Design review of the part built by this model. Coordinates are the model's own, in mm. Round coordinates to 2 decimals unless told otherwise and drop trailing zeros. One line per item, written item: value. Start each with the question number.
Item 1: For line 1 along Y through (x, z) = (-16.75, 168.5); line 2 along Y through (x, z) = (-12.7, 100.5); line 3 along X through (y, z) = (11, 50), list the stretches that pass through material, from the lowest coordinate up.
Item 2: Clearance check with flat-ended pins moving along their axes: pin 1 (3 mm diameter, centred on x = -12.5, z = 71, fed in from -Y); pin 2 (1.5 mm diameter, centred on y = 12, z = 160, fed in from +X); pin 3 (1.5 mm diameter, centred on y = 12.5, z = 79, fed in from -X). State where each tip first meets the part, or that it passes through.
Item 3: Mouldability with a two-part tool opening along X and no side actions: class faces 1 (the cylindrical face through (-1.086, 24.254, 106.439)), 2 (the cylindrical face through (-15.18, 14.97, 106.44)), 3 (the flat face through (-16, 16, 215.9)), 4 (the flat face through (-25.4, 19, 106)) as released by +X, released by -X, zero draft, split by the parting line, or undercut.
from build123d import *

# Parameters (mm, degrees)
F0_R     = 3.362501
F1_DEPTH = 215.9


with BuildPart() as f1:
    # F0 (on Top) → F1 (new body)
    with BuildSketch(Plane.XY):
        with BuildLine():
            ThreePointArc((-8.548576, 18.755238), (-9.784629, 17.929334), (-11.242653, 17.639315))
            Line((-11.242653, 17.639315), (-14.157347, 17.639315))
            ThreePointArc((-14.157347, 17.639315), (-15.615371, 17.929334), (-16.851424, 18.755238))
            Line((-16.851424, 18.755238), (-18.696905, 20.600719))
            ThreePointArc((-18.696905, 20.600719), (-19.109857, 22.67677), (-17.349867, 23.852758))
            Line((-17.349867, 23.852758), (-15.615371, 23.852758))
            Line((-15.615371, 23.852758), (-15.58302, 23.852758))
            ThreePointArc((-15.58302, 23.852758), (-14.825405, 24.626379), (-15.58302, 25.4))
            Line((-15.58302, 25.4), (-15.615371, 25.4))
            Line((-15.615371, 25.4), (-16.253341, 25.4))
            ThreePointArc((-16.253341, 25.4), (-16.801604, 24.858772), (-17.349867, 25.4))
            Line((-17.349867, 25.4), (-20.487482, 25.4))
            ThreePointArc((-20.487482, 25.4), (-21.038741, 24.848741), (-21.59, 25.4))
            ThreePointArc((-21.59, 25.4), (-24.284077, 24.284077), (-25.4, 21.59))
            Line((-25.4, 21.59), (-25.4, 20.504724))
            Line((-25.4, 20.504724), (-25.4, 17.349867))
            ThreePointArc((-25.4, 17.349867), (-24.844161, 16.802675), (-25.4, 16.255483))
            Line((-25.4, 16.255483), (-25.4, 15.615371))
            ThreePointArc((-25.4, 15.615371), (-24.626379, 14.859554), (-23.852758, 15.615371))
            Line((-23.852758, 15.615371), (-23.852758, 17.349867))
            ThreePointArc((-23.852758, 17.349867), (-22.67677, 19.109857), (-20.600719, 18.696905))
            Line((-20.600719, 18.696905), (-18.755238, 16.851424))
            ThreePointArc((-18.755238, 16.851424), (-17.929334, 15.615371), (-17.639315, 14.157347))
            Line((-17.639315, 14.157347), (-17.639315, 11.242653))
            ThreePointArc((-17.639315, 11.242653), (-17.929334, 9.784629), (-18.755238, 8.548576))
            Line((-18.755238, 8.548576), (-20.600719, 6.703095))
            ThreePointArc((-20.600719, 6.703095), (-22.67677, 6.290143), (-23.852758, 8.050133))
            Line((-23.852758, 8.050133), (-23.852758, 9.784629))
            ThreePointArc((-23.852758, 9.784629), (-24.626379, 10.55825), (-25.4, 9.784629))
            Line((-25.4, 9.784629), (-25.4, 9.149239))
            ThreePointArc((-25.4, 9.149239), (-24.899374, 8.599686), (-25.4, 8.050133))
            Line((-25.4, 8.050133), (-25.4, 4.904538))
            ThreePointArc((-25.4, 4.904538), (-24.846216, 4.357269), (-25.4, 3.81))
            ThreePointArc((-25.4, 3.81), (-24.284077, 1.115923), (-21.59, 0))
            ThreePointArc((-21.59, 0), (-21.040817, 0.554885), (-20.491634, 0))
            Line((-20.491634, 0), (-16.708169, 0))
            ThreePointArc((-16.708169, 0), (-16.16177, 0.540135), (-15.615371, 0))
            ThreePointArc((-15.615371, 0), (-14.854184, 0.7747), (-15.615371, 1.5494))
            Line((-15.615371, 1.5494), (-17.347709, 1.5494))
            ThreePointArc((-17.347709, 1.5494), (-19.107699, 2.725388), (-18.694747, 4.801438))
            Line((-18.694747, 4.801438), (-16.851424, 6.644762))
            ThreePointArc((-16.851424, 6.644762), (-15.615371, 7.470666), (-14.157347, 7.760685))
            Line((-14.157347, 7.760685), (-11.242653, 7.760685))
            ThreePointArc((-11.242653, 7.760685), (-9.784629, 7.470666), (-8.548576, 6.644762))
            Line((-8.548576, 6.644762), (-6.705253, 4.801438))
            ThreePointArc((-6.705253, 4.801438), (-6.292301, 2.725388), (-8.052291, 1.5494))
            Line((-8.052291, 1.5494), (-9.784629, 1.5494))
            ThreePointArc((-9.784629, 1.5494), (-10.401836, 0.7747), (-9.784629, 0))
            Line((-9.784629, 0), (-9.152868, 0))
            ThreePointArc((-9.152868, 0), (-8.602579, 0.545262), (-8.052291, 0))
            Line((-8.052291, 0), (-4.898866, 0))
            ThreePointArc((-4.898866, 0), (-4.354433, 0.544433), (-3.81, 0))
            ThreePointArc((-3.81, 0), (-1.115923, 1.115923), (0, 3.81))
            ThreePointArc((0, 3.81), (-0.53938, 4.3561), (0, 4.9022))
            Line((0, 4.9022), (0, 8.052291))
            ThreePointArc((0, 8.052291), (-0.543517, 8.60166), (0, 9.151029))
            Line((0, 9.151029), (0, 9.784629))
            ThreePointArc((0, 9.784629), (-0.7747, 10.504691), (-1.5494, 9.784629))
            Line((-1.5494, 9.784629), (-1.5494, 8.052291))
            ThreePointArc((-1.5494, 8.052291), (-2.725388, 6.292301), (-4.801438, 6.705253))
            Line((-4.801438, 6.705253), (-6.644762, 8.548576))
            ThreePointArc((-6.644762, 8.548576), (-7.470666, 9.784629), (-7.760685, 11.242653))
            Line((-7.760685, 11.242653), (-7.760685, 14.157347))
            ThreePointArc((-7.760685, 14.157347), (-7.470666, 15.615371), (-6.644762, 16.851424))
            Line((-6.644762, 16.851424), (-4.801438, 18.694747))
            ThreePointArc((-4.801438, 18.694747), (-2.725388, 19.107699), (-1.5494, 17.347709))
            Line((-1.5494, 17.347709), (-1.5494, 15.615371))
            ThreePointArc((-1.5494, 15.615371), (-0.7747, 14.879405), (0, 15.615371))
            Line((0, 15.615371), (0, 16.255509))
            ThreePointArc((0, 16.255509), (-0.5461, 16.801609), (0, 17.347709))
            Line((0, 17.347709), (0, 20.495165))
            ThreePointArc((0, 20.495165), (-0.551056, 21.042583), (0, 21.59))
            ThreePointArc((0, 21.59), (-1.115923, 24.284077), (-3.81, 25.4))
            ThreePointArc((-3.81, 25.4), (-4.365303, 24.903619), (-4.920606, 25.4))
            Line((-4.920606, 25.4), (-8.050133, 25.4))
            ThreePointArc((-8.050133, 25.4), (-8.596365, 24.859433), (-9.142596, 25.4))
            Line((-9.142596, 25.4), (-9.784629, 25.4))
            Line((-9.784629, 25.4), (-9.856203, 25.4))
            ThreePointArc((-9.856203, 25.4), (-10.594864, 24.626379), (-9.856203, 23.852758))
            Line((-9.856203, 23.852758), (-9.784629, 23.852758))
            Line((-9.784629, 23.852758), (-8.050133, 23.852758))
            ThreePointArc((-8.050133, 23.852758), (-6.290143, 22.67677), (-6.703095, 20.600719))
            Line((-6.703095, 20.600719), (-8.548576, 18.755238))
        make_face()
        with Locations((-12.7, 12.7)):
            Circle(F0_R, mode=Mode.SUBTRACT)
        with BuildLine():
            ThreePointArc((-9.856203, 23.852758), (-9.820416, 23.851931), (-9.784629, 23.852758))
            Line((-9.784629, 23.852758), (-9.856203, 23.852758))
        make_face()
        with BuildLine():
            Line((-15.58302, 23.852758), (-15.615371, 23.852758))
            ThreePointArc((-15.615371, 23.852758), (-15.599195, 23.852589), (-15.58302, 23.852758))
        make_face()
        with BuildLine():
            ThreePointArc((-9.784629, 25.4), (-9.820416, 25.400827), (-9.856203, 25.4))
            Line((-9.856203, 25.4), (-9.784629, 25.4))
        make_face()
        with BuildLine():
            Line((-15.615371, 25.4), (-15.58302, 25.4))
            ThreePointArc((-15.58302, 25.4), (-15.599195, 25.400169), (-15.615371, 25.4))
        make_face()
    extrude(amount=F1_DEPTH)


solid = f1.part
A:
1. line 1: 0 to 1.55, 6.74 to 18.66, 23.85 to 24.86
1. line 2: 7.76 to 9.34, 16.06 to 17.64
1. line 3: -17.65 to -15.6, -9.8 to -7.75
2. pin 1: y = 7.75
2. pin 2: x = -7.76
2. pin 3: x = -17.64
3. face 1: released by +X
3. face 2: undercut
3. face 3: zero draft
3. face 4: released by -X
